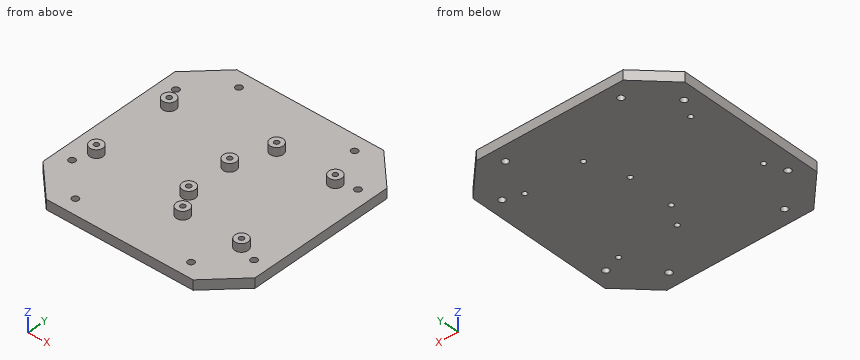
from build123d import *

# Parameters (mm, degrees)
SKETCH_1_W          = 130
SKETCH_1_H          = 130
EXTRUDE_1_DEPTH     = 6
SKETCH_10_R         = 1.5
CUT_EXTRUDE_1_DEPTH = 6
CUT_EXTRUDE_2_REACH = 185.946
SKETCH_11_R         = 2
CHAMFER_1_SIZE      = 20
CUT_EXTRUDE_3_REACH = 185.946
SKETCH_12_R         = 1.5
EXTRUDE_START       = 5
SKETCH_13_R         = 4
SKETCH_13_R_2       = 1.5
EXTRUDE_2_DEPTH     = 5


with BuildPart() as part:
    # 草圖1 → 填料-伸長1 (new body)
    with BuildSketch(Plane.XY):
        with Locations((-65, 65)):
            Rectangle(SKETCH_1_W, SKETCH_1_H)
    extrude(amount=EXTRUDE_1_DEPTH)

    # 草圖10 → 除料-伸長1 (cut)
    with BuildSketch(Plane.XY.offset(6)):
        with Locations((-114.76, 89.13)):
            Circle(SKETCH_10_R)
        with Locations((-63.96, 73.89)):
            Circle(SKETCH_10_R)
        with Locations((-63.96, 45.95)):
            Circle(SKETCH_10_R)
        with Locations((-116.03, 40.87)):
            Circle(SKETCH_10_R)
    extrude(amount=-CUT_EXTRUDE_1_DEPTH, mode=Mode.SUBTRACT)

    # 草圖11 → 除料-伸長2 (cut, up to next)
    with BuildSketch(Plane.XY.offset(6), mode=Mode.PRIVATE) as cut_extrude_2_sk1:
        with Locations((-9.2, 100.435324702)):
            Circle(SKETCH_11_R)
    cut_extrude_2_tool1 = extrude(cut_extrude_2_sk1.sketch, amount=-CUT_EXTRUDE_2_REACH, mode=Mode.PRIVATE) & part.part
    # 草圖11 → 除料-伸長2 (cut, up to next)
    with BuildSketch(Plane.XY.offset(6), mode=Mode.PRIVATE) as cut_extrude_2_sk2:
        with Locations((-29.564675298, 120.8)):
            Circle(SKETCH_11_R)
    cut_extrude_2_tool2 = extrude(cut_extrude_2_sk2.sketch, amount=-CUT_EXTRUDE_2_REACH, mode=Mode.PRIVATE) & part.part
    # 草圖11 → 除料-伸長2 (cut, up to next)
    with BuildSketch(Plane.XY.offset(6), mode=Mode.PRIVATE) as cut_extrude_2_sk3:
        with Locations((-100.435324702, 120.8)):
            Circle(SKETCH_11_R)
    cut_extrude_2_tool3 = extrude(cut_extrude_2_sk3.sketch, amount=-CUT_EXTRUDE_2_REACH, mode=Mode.PRIVATE) & part.part
    # 草圖11 → 除料-伸長2 (cut, up to next)
    with BuildSketch(Plane.XY.offset(6), mode=Mode.PRIVATE) as cut_extrude_2_sk4:
        with Locations((-120.8, 100.435324702)):
            Circle(SKETCH_11_R)
    cut_extrude_2_tool4 = extrude(cut_extrude_2_sk4.sketch, amount=-CUT_EXTRUDE_2_REACH, mode=Mode.PRIVATE) & part.part
    # 草圖11 → 除料-伸長2 (cut, up to next)
    with BuildSketch(Plane.XY.offset(6), mode=Mode.PRIVATE) as cut_extrude_2_sk5:
        with Locations((-120.8, 29.564675298)):
            Circle(SKETCH_11_R)
    cut_extrude_2_tool5 = extrude(cut_extrude_2_sk5.sketch, amount=-CUT_EXTRUDE_2_REACH, mode=Mode.PRIVATE) & part.part
    # 草圖11 → 除料-伸長2 (cut, up to next)
    with BuildSketch(Plane.XY.offset(6), mode=Mode.PRIVATE) as cut_extrude_2_sk6:
        with Locations((-100.435324702, 9.2)):
            Circle(SKETCH_11_R)
    cut_extrude_2_tool6 = extrude(cut_extrude_2_sk6.sketch, amount=-CUT_EXTRUDE_2_REACH, mode=Mode.PRIVATE) & part.part
    # 草圖11 → 除料-伸長2 (cut, up to next)
    with BuildSketch(Plane.XY.offset(6), mode=Mode.PRIVATE) as cut_extrude_2_sk7:
        with Locations((-29.564675298, 9.2)):
            Circle(SKETCH_11_R)
    cut_extrude_2_tool7 = extrude(cut_extrude_2_sk7.sketch, amount=-CUT_EXTRUDE_2_REACH, mode=Mode.PRIVATE) & part.part
    # 草圖11 → 除料-伸長2 (cut, up to next)
    with BuildSketch(Plane.XY.offset(6), mode=Mode.PRIVATE) as cut_extrude_2_sk8:
        with Locations((-9.2, 29.564675298)):
            Circle(SKETCH_11_R)
    cut_extrude_2_tool8 = extrude(cut_extrude_2_sk8.sketch, amount=-CUT_EXTRUDE_2_REACH, mode=Mode.PRIVATE) & part.part
    add(cut_extrude_2_tool1.solids().sort_by_distance((-9.2, 100.435325, 6))[0], mode=Mode.SUBTRACT)
    add(cut_extrude_2_tool2.solids().sort_by_distance((-29.564675, 120.8, 6))[0], mode=Mode.SUBTRACT)
    add(cut_extrude_2_tool3.solids().sort_by_distance((-100.435325, 120.8, 6))[0], mode=Mode.SUBTRACT)
    add(cut_extrude_2_tool4.solids().sort_by_distance((-120.8, 100.435325, 6))[0], mode=Mode.SUBTRACT)
    add(cut_extrude_2_tool5.solids().sort_by_distance((-120.8, 29.564675, 6))[0], mode=Mode.SUBTRACT)
    add(cut_extrude_2_tool6.solids().sort_by_distance((-100.435325, 9.2, 6))[0], mode=Mode.SUBTRACT)
    add(cut_extrude_2_tool7.solids().sort_by_distance((-29.564675, 9.2, 6))[0], mode=Mode.SUBTRACT)
    add(cut_extrude_2_tool8.solids().sort_by_distance((-9.2, 29.564675, 6))[0], mode=Mode.SUBTRACT)

    # 導角1
    chamfer_1_edges = [part.edges().sort_by_distance(p)[0] for p in [
        (-130, 0, 3),
        (-130, 130, 3),
        (0, 130, 3),
        (0, 0, 3),
    ]]
    chamfer(chamfer_1_edges, length=CHAMFER_1_SIZE)

    # 草圖12 → 除料-伸長3 (cut, up to next)
    with BuildSketch(Plane.XY.offset(6), mode=Mode.PRIVATE) as cut_extrude_3_sk1:
        with Locations((-56, 97)):
            Circle(SKETCH_12_R)
    cut_extrude_3_tool1 = extrude(cut_extrude_3_sk1.sketch, amount=-CUT_EXTRUDE_3_REACH, mode=Mode.PRIVATE) & part.part
    # 草圖12 → 除料-伸長3 (cut, up to next)
    with BuildSketch(Plane.XY.offset(6), mode=Mode.PRIVATE) as cut_extrude_3_sk2:
        with Locations((-20, 97)):
            Circle(SKETCH_12_R)
    cut_extrude_3_tool2 = extrude(cut_extrude_3_sk2.sketch, amount=-CUT_EXTRUDE_3_REACH, mode=Mode.PRIVATE) & part.part
    # 草圖12 → 除料-伸長3 (cut, up to next)
    with BuildSketch(Plane.XY.offset(6), mode=Mode.PRIVATE) as cut_extrude_3_sk3:
        with Locations((-56, 33)):
            Circle(SKETCH_12_R)
    cut_extrude_3_tool3 = extrude(cut_extrude_3_sk3.sketch, amount=-CUT_EXTRUDE_3_REACH, mode=Mode.PRIVATE) & part.part
    # 草圖12 → 除料-伸長3 (cut, up to next)
    with BuildSketch(Plane.XY.offset(6), mode=Mode.PRIVATE) as cut_extrude_3_sk4:
        with Locations((-20, 33)):
            Circle(SKETCH_12_R)
    cut_extrude_3_tool4 = extrude(cut_extrude_3_sk4.sketch, amount=-CUT_EXTRUDE_3_REACH, mode=Mode.PRIVATE) & part.part
    add(cut_extrude_3_tool1.solids().sort_by_distance((-56, 97, 6))[0], mode=Mode.SUBTRACT)
    add(cut_extrude_3_tool2.solids().sort_by_distance((-20, 97, 6))[0], mode=Mode.SUBTRACT)
    add(cut_extrude_3_tool3.solids().sort_by_distance((-56, 33, 6))[0], mode=Mode.SUBTRACT)
    add(cut_extrude_3_tool4.solids().sort_by_distance((-20, 33, 6))[0], mode=Mode.SUBTRACT)

    # 草圖13 → 填料-伸長2 (add)
    # profile 1 of 8: a face of its own
    with BuildSketch(Plane.XY.offset(6).offset(EXTRUDE_START)):
        with Locations((-114.76, 89.13)):
            Circle(SKETCH_13_R)
        with Locations((-114.76, 89.13)):
            Circle(SKETCH_13_R_2, mode=Mode.SUBTRACT)
    # profile 2 of 8: a face of its own
    with BuildSketch(Plane.XY.offset(6).offset(EXTRUDE_START)):
        with Locations((-56, 97)):
            Circle(SKETCH_13_R)
        with Locations((-56, 97)):
            Circle(SKETCH_13_R_2, mode=Mode.SUBTRACT)
    # profile 3 of 8: a face of its own
    with BuildSketch(Plane.XY.offset(6).offset(EXTRUDE_START)):
        with Locations((-116.03, 40.87)):
            Circle(SKETCH_13_R)
        with Locations((-116.03, 40.87)):
            Circle(SKETCH_13_R_2, mode=Mode.SUBTRACT)
    # profile 4 of 8: a face of its own
    with BuildSketch(Plane.XY.offset(6).offset(EXTRUDE_START)):
        with Locations((-63.96, 73.89)):
            Circle(SKETCH_13_R)
        with Locations((-63.96, 73.89)):
            Circle(SKETCH_13_R_2, mode=Mode.SUBTRACT)
    # profile 5 of 8: a face of its own
    with BuildSketch(Plane.XY.offset(6).offset(EXTRUDE_START)):
        with Locations((-63.96, 45.95)):
            Circle(SKETCH_13_R)
        with Locations((-63.96, 45.95)):
            Circle(SKETCH_13_R_2, mode=Mode.SUBTRACT)
    # profile 6 of 8: a face of its own
    with BuildSketch(Plane.XY.offset(6).offset(EXTRUDE_START)):
        with Locations((-56, 33)):
            Circle(SKETCH_13_R)
        with Locations((-56, 33)):
            Circle(SKETCH_13_R_2, mode=Mode.SUBTRACT)
    # profile 7 of 8: a face of its own
    with BuildSketch(Plane.XY.offset(6).offset(EXTRUDE_START)):
        with Locations((-20, 33)):
            Circle(SKETCH_13_R)
        with Locations((-20, 33)):
            Circle(SKETCH_13_R_2, mode=Mode.SUBTRACT)
    # profile 8 of 8: a face of its own
    with BuildSketch(Plane.XY.offset(6).offset(EXTRUDE_START)):
        with Locations((-20, 97)):
            Circle(SKETCH_13_R)
        with Locations((-20, 97)):
            Circle(SKETCH_13_R_2, mode=Mode.SUBTRACT)
    extrude(amount=-EXTRUDE_2_DEPTH)


solid = part.part
Read the model definition and answer for the solid it produces. Units are mm, in the model's axes. Round coordinates to 2 decimals unless told otherwise and drop trailing zeros. Order: outer loops, then holes, each group sorted by start corner. A loop starts at its lowest first (then second) coordinate and runs counter-clockwise, first axis right, second up.
1) The part is cut by section C-C on y = 120.8. Write down the section's boundary in (x, z), plus the area to 3 significant figures.
2) The part is cut by section D-D on z = 4.5. Give the number of separate pieces and of enclosed holes in the cut face, plus the area to 3 significant figures.
3) The part is cut by section B-B on y = 89.13. Write down the section's boundary in (x, z), plus the area to 3 significant figures.
4) Straight lines are drawn through the part: L1, parallel to Y at x = -63.96, z = 3; L2, parallel to Y at x = -20, z = 2.5; L3, parallel to X at y = 97, z = 5.5. For each, find the intervals that lie inside material, in ascending order.
5) Flat-ended cylindrical pins translate along their axes: pin 1 (2 mm diameter, centred on x = -65, z = 9.5, fed in from -Y); pin 2 (2 mm diameter, centred on x = -98.5, y = 74.5, fed in from +Z); pin 3 (1.5 mm diameter, centred on y = 14.5, z = 2.5, fed in from +X). Find the tip coordinate at first contact, or state that the pin passes through.
6) The part is cut by section A-A on x = -56. Write down the section's boundary in (y, z).
Resolved:
1. outline: (-119.2, 0) - (-102.44, 0) - (-102.44, 6) - (-119.2, 6) - close; (-98.44, 0) - (-31.56, 0) - (-31.56, 6) - (-98.44, 6) - close; (-27.56, 0) - (-10.8, 0) - (-10.8, 6) - (-27.56, 6) - close
1. area: 602 mm2
2. separate pieces: 1
2. enclosed holes: 16
2. area: 15,900 mm2
3. outline: (-130, 0) - (-116.26, 0) - (-116.26, 11) - (-118.76, 11) - (-118.76, 6) - (-130, 6) - close; (-113.26, 0) - (0, 0) - (0, 6) - (-110.76, 6) - (-110.76, 11) - (-113.26, 11) - close
3. area: 787 mm2
4. L1: y = 0 to 44.45, 47.45 to 72.39, 75.39 to 130
4. L2: y = 0 to 31.5, 34.5 to 95.5, 98.5 to 130
4. L3: x = -130 to -57.5, -54.5 to -21.5, -18.5 to 0
5. pin 1: stops at y = 41.95
5. pin 2: stops at z = 6
5. pin 3: stops at x = -4.75
6. outline: (0, 0) - (31.5, 0) - (31.5, 11) - (29, 11) - (29, 6) - (0, 6) - close; (34.5, 0) - (95.5, 0) - (95.5, 11) - (93, 11) - (93, 6) - (37, 6) - (37, 11) - (34.5, 11) - close; (98.5, 0) - (130, 0) - (130, 6) - (101, 6) - (101, 11) - (98.5, 11) - close
